Read the model definition and answer for the solid it produces. Units are mm, in the model's axes. Face numbers are marked on the shaded views. Give positions to 0.01 mm unless a question says otherwise; leave off trailing zeros. Write each loop counter-clockwise with the first axis right and the second up, starting at its lowest first coordinate (ties: lowest second). Pieces come first, ordered by that corner, then holes.
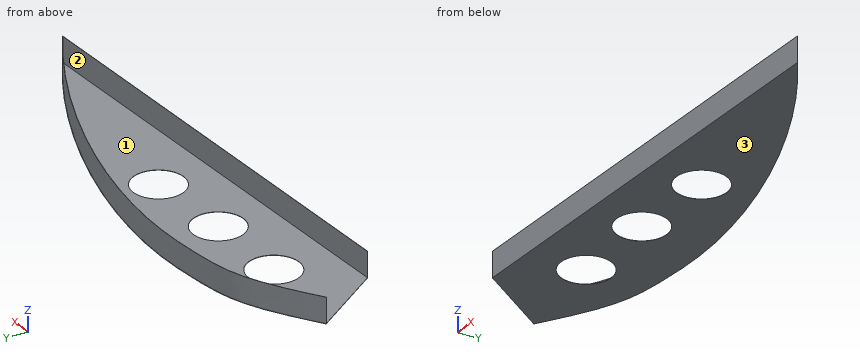
```python
from build123d import *

# Parameters (mm, degrees)
SKETCH1_R           = 10
BOSS_EXTRUDE1_DEPTH = 0.1
BOSS_EXTRUDE2_DEPTH = 10
BOSS_EXTRUDE5_DEPTH = 10


with BuildPart() as part:
    # Sketch1 → Boss-Extrude1 (new body)
    with BuildSketch(Plane.XY):
        with BuildLine():
            Line((-1743.607960183, 593.830470178), (-1723.97557604, 565.354199265))
            Line((-1723.97557604, 565.354199265), (-1544.649956659, 573.44143308))
            add(Edge.make_bspline(
                [(-1743.607960183, 593.830470178), (-1719.507904213, 610.537812828), (-1709.389541143, 613.399774739), (-1646.280289738, 619.241808081), (-1585.716648888, 600.423930323), (-1544.649956659, 573.44143308)],
                knots=[0, 0, 0, 0, 0.320554642, 0.420554642, 1, 1, 1, 1], degree=3))
        make_face()
        with Locations((-1632.906290904, 590.670757295)):
            Circle(SKETCH1_R, mode=Mode.SUBTRACT)
        with Locations((-1667.865738011, 588.986400452)):
            Circle(SKETCH1_R, mode=Mode.SUBTRACT)
        with Locations((-1702.865738011, 588.986400452)):
            Circle(SKETCH1_R, mode=Mode.SUBTRACT)
    extrude(amount=BOSS_EXTRUDE1_DEPTH)

    # Sketch2 → Boss-Extrude2 (add)
    with BuildSketch(Plane.XY.offset(0.1)):
        Polygon((-1724.027783053, 565.451946471), (-1723.97557604, 565.354199265), (-1544.79832648, 573.434741892), (-1544.802831705, 573.534640355), align=None)
    extrude(amount=BOSS_EXTRUDE2_DEPTH)

    # Sketch3 → Boss-Extrude5 (add)
    with BuildSketch(Plane.XY.offset(0.1)):
        with BuildLine():
            Line((-1545.023079711, 573.566578824), (-1545.182742706, 573.5515561))
            add(Edge.make_bspline(
                [(-1545.182742706, 573.5515561), (-1547.367111706, 574.980268212), (-1551.810044118, 577.785328256), (-1560.965598012, 583.174479228), (-1572.795764, 589.430500324), (-1587.376218754, 596.094131565), (-1607.088908765, 603.794197945), (-1626.860275971, 609.633108879), (-1645.984019518, 613.443251497), (-1659.830715168, 615.239913168), (-1672.989792243, 615.951202382), (-1683.282773373, 615.549802626), (-1690.803354798, 614.881158472), (-1697.680820628, 614.1264693), (-1704.980899474, 613.117091179), (-1711.55998554, 611.460964287), (-1716.962589709, 609.43710742), (-1721.23073898, 607.488971473), (-1725.859262309, 605.030940979), (-1730.13578168, 602.491531609), (-1733.880880623, 600.125360581), (-1736.867805363, 598.174714985), (-1739.526085034, 596.39020329), (-1741.749970087, 594.871411779), (-1742.918244581, 594.065255562), (-1743.494013607, 593.66610419)],
                knots=[0.001987871, 0.001987871, 0.001987871, 0.001987871, 0.032699504, 0.063902746, 0.126309229, 0.188715713, 0.251122197, 0.375935164, 0.438341647, 0.500748131, 0.563154615, 0.625561098, 0.65676434, 0.687967582, 0.750374066, 0.812780549, 0.843983791, 0.875187033, 0.906390275, 0.937593516, 0.953195137, 0.968796758, 0.984398379, 0.99219919, 1, 1, 1, 1], degree=3))
            Line((-1743.494013607, 593.66610419), (-1743.550986895, 593.748287184))
            add(Edge.make_bspline(
                [(-1545.023079711, 573.566578824), (-1580.385570882, 596.721777486), (-1623.540098869, 611.77846709), (-1664.058944494, 615.565415197), (-1668.460623745, 615.803565887), (-1674.850272895, 615.874635067), (-1676.946082289, 615.848904453), (-1681.051562144, 615.71013567), (-1685.067312648, 615.488156686), (-1688.83699666, 615.1571463), (-1692.450372149, 614.800321889), (-1694.177045989, 614.610346383), (-1699.085739343, 614.035305054), (-1702.019101267, 613.629485697), (-1710.378502815, 612.027658053), (-1715.364224243, 610.448022257), (-1727.252760657, 604.56560412), (-1734.155086468, 600.261986909), (-1743.550986895, 593.748287184)],
                knots=[0.001496262, 0.001496262, 0.001496262, 0.001496262, 0.5, 0.5, 0.5625, 0.5625, 0.59375, 0.59375, 0.625, 0.65625, 0.65625, 0.6875, 0.6875, 0.75, 0.75, 0.875, 0.875, 1, 1, 1, 1], degree=3))
        make_face()
    extrude(amount=BOSS_EXTRUDE5_DEPTH)


solid = part.part
```
Item 1: Each of these flat-tipped pins is pushed along its axis until it touches: pin 1 Ø6 at (x, z) = (-1606.5, 6) entering from +Y; pin 2 Ø6 at (x, z) = (-1712, 3.5) entering from -Y; pin 3 Ø2 at (x, y) = (-1664, 576.5) entering from +Z; pin 4 Ø12 at (x, y) = (-1696, 608) entering from -Z. Where does it stop, or does it pass through?
Result set:
pin 1: stops at y = 604.34
pin 2: stops at y = 565.76
pin 3: stops at z = 0.1
pin 4: stops at z = 0
Item 2: Section B-B (y = 584) is taken. Give the number of separate pieces and of enclosed holes in the cut face, and give its area (3 significant figures).
Result set:
separate pieces: 4
enclosed holes: 0
area: 14.6 mm2
Item 3: Determine the mould class of the marked faces 1, 2 and 3 for opening direction X: pulls with the +X half, pulls with the -X half, needs draft (parallel to the pull), parting line crosses it, or undercut.
Result set:
face 1: undercut
face 2: pulls with the -X half
face 3: needs draft
Item 4: Find the intervals of material crossed by line 1 along X through (y, z) = (594.5, 0.75); line 2 along X through (y, z) = (577.5, 3.5); line 3 along X through (y, z) = (581, 9), in increasing order.
Result set:
line 1: x = -1742.46 to -1742.29, -1584.06 to -1583.81
line 2: x = -1551.42 to -1551.23
line 3: x = -1557.31 to -1557.11
Item 5: Section A-A (y = 570) is taken. Write down the section's boundary in (x, z), and give its area (3 significant figures).
Result set:
outline: (-1727.18, 0) - (-1620.96, 0) - (-1620.96, 10.1) - (-1623.18, 10.1) - (-1623.18, 0.1) - (-1727.18, 0.1) - close
area: 32.8 mm2
